Here's how the part is built. I have some questions about the finished solid (model axes, mm). Face numbers are marked on the shaded views. A direction names the side the tool comes from. Give positions to 0.01 mm unless a question says otherwise; leave off trailing zeros. Write each loop counter-clockwise with the first axis right and the second up, starting at its lowest first coordinate (ties: lowest second). Pieces come first, ordered by that corner, then holes. Notation, with made-up numbers: M 39.5,52.25 L 72.5,52.25 A17 ccw 72.5,73.25 Z; hole C -23,23 d2. An arc over 180 degrees is marked long. Answer as CSV lines item,"result". Start each with the question number.
Q1. Suppose I cut it at D-D (z = 5). Write out the boundary of the cut face in (x, y).
Q2. Suppose I cut it at A-A (y = -0.2). Write out the boundary of the cut face in (x, z) (3 decimals).
Q3. Suppose I cut it at B-B (x = -4). Write out the boundary of the cut face in (y, z), then the cut area to 3 significant figures.
Q4. For pin 1 (0.8 mm diameter, centred on x = 0.5, z = 2.5, fed in from -Y); pin 2 (3 mm diameter, centred on y = 5, z = 2.5, fed in from +X) (3 decimals); pin 3 (1.4 mm diameter, centred on y = 6.5, z = 2, fed in from -X) (3 decimals); pin 4 (1.8 mm diameter, centred on x = 10.775, y = -0.2, fed in from -Z), each with a flat end and sliding along its axis, tell me the tip position at first contact or that it passes through.
Q5. If I drill on line 1 along Y through (x, z) = (-2.5, 2); line 2 along Z through (x, y) = (4.25, 7.25); line 3 along Y through (x, z) = (10.25, 0.5), over which ranges is the centre line in solid material (lowest first)?
Q6. Suppose I cut it at C-C (y = -10.75). Write out the boundary of the cut face in (x, z) (3 decimals).
Q7. On a 3-axis mill with a long thin cutter (end or side, diameter ignored), from which of +Z, -Z, +X, -X, +Y, -Y can I reach the whole of each face in a straight line? I mean the marked faces 4, 5, 6 and 7. Say none if no direction works.
Q8. Thinking about a two-plate mould opening in Y: for the marked faces 1, 2 and 3, which applies, +Y half, -Y half, draft (parallel to the pull), parting line (faces both ways), or undercut?
```python
from build123d import *

# Parameters (mm, degrees)
F0_W     = 25.75
F0_H     = 28.3
F0_W_2   = 15.1
F0_H_2   = 9.6
F0_R     = 1
F0_W_3   = 20.85
F0_H_3   = 7
F1_DEPTH = 1.15
F2_DEPTH = 3.9
F3_DEPTH = 7.35


with BuildPart() as f1:
    # F0 (on Top) → F1 (new body)
    with BuildSketch(Plane.XY):
        Rectangle(F0_W, F0_H)
        with Locations((0, -8.35)):
            Rectangle(F0_W_2, F0_H_2, mode=Mode.SUBTRACT)
        with Locations((-10.775, -0.2)):
            Circle(F0_R, mode=Mode.SUBTRACT)
        with Locations((10.775, -0.2)):
            Circle(F0_R, mode=Mode.SUBTRACT)
        with Locations((0, 5.65)):
            Rectangle(F0_W_3, F0_H_3, mode=Mode.SUBTRACT)
        with Locations((-10.775, 12.05)):
            Circle(F0_R, mode=Mode.SUBTRACT)
        with Locations((10.775, 12.05)):
            Circle(F0_R, mode=Mode.SUBTRACT)
    extrude(amount=F1_DEPTH)

    # F0 (on Top) → F2 (join)
    with BuildSketch(Plane.XY):
        with Locations((0, 5.65)):
            Rectangle(F0_W_3, F0_H_3)
    extrude(amount=F2_DEPTH)

    # F0 (on Top) → F3 (join)
    with BuildSketch(Plane.XY):
        with Locations((0, -8.35)):
            Rectangle(F0_W_2, F0_H_2)
    extrude(amount=F3_DEPTH)


solid = f1.part
```
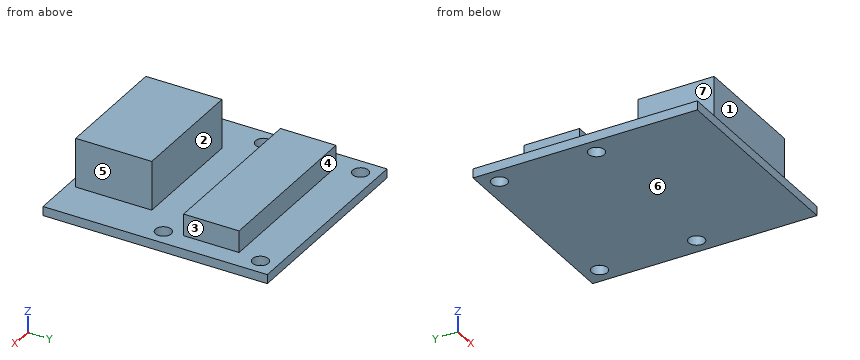
Resolved:
1,outline,"M -7.55,-13.15 L 7.55,-13.15 L 7.55,-3.55 L -7.55,-3.55 Z"
2,outline,"M -12.875,0 L -11.775,0 L -11.775,1.15 L -12.875,1.15 Z; M -9.775,0 L 9.775,0 L 9.775,1.15 L -9.775,1.15 Z; M 11.775,0 L 12.875,0 L 12.875,1.15 L 11.775,1.15 Z"
3,outline,"M -14.15,0 L 14.15,0 L 14.15,1.15 L 9.15,1.15 L 9.15,3.9 L 2.15,3.9 L 2.15,1.15 L -3.55,1.15 L -3.55,7.35 L -13.15,7.35 L -13.15,1.15 L -14.15,1.15 Z"
3,area,"111 mm^2"
4,pin 1,"y = -13.15"
4,pin 2,"x = 12.875"
4,pin 3,"x = -10.425"
4,pin 4,"through"
5,line 1,"-13.15 to -3.55, 2.15 to 9.15"
5,line 2,"0 to 3.9"
5,line 3,"-14.15 to -1.05, 0.65 to 11.2, 12.9 to 14.15"
6,outline,"M -12.875,0 L 12.875,0 L 12.875,1.15 L 7.55,1.15 L 7.55,7.35 L -7.55,7.35 L -7.55,1.15 L -12.875,1.15 Z"
7,face 4,"+Z, +X, -X, +Y"
7,face 5,"+Z, +X, -Y"
7,face 6,"-Z, +X, -X, +Y, -Y"
7,face 7,"+Z, -X, -Y"
8,face 1,"-Y half"
8,face 2,"undercut"
8,face 3,"draft"
